Model file for the job. Use its own axes, mm. Face numbers are marked on the shaded views. Give positions to 0.01 mm unless a question says otherwise; leave off trailing zeros. Write each loop counter-clockwise with the first axis right and the second up, starting at its lowest first coordinate (ties: lowest second). Pieces come first, ordered by that corner, then holes.
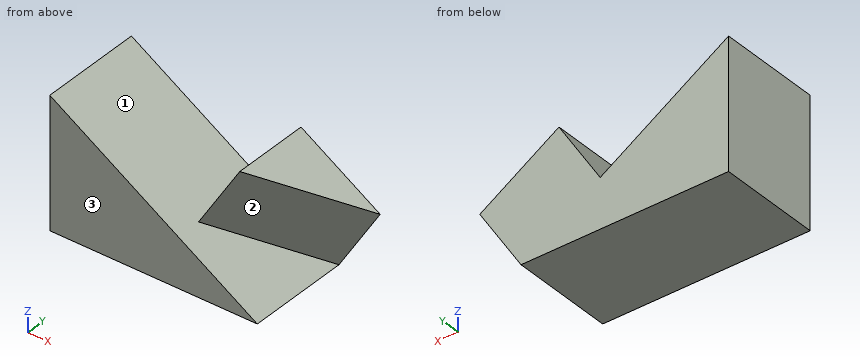
```python
from build123d import *

# Parameters (mm, degrees)
F1_DEPTH = 25.4
F3_DEPTH = 19.05


with BuildPart() as f1:
    # F0 (on Front) → F1 (new body)
    with BuildSketch(Plane.XZ):
        Polygon((0, 31.75), (0, 0), (50.8, 0), align=None)
    extrude(amount=F1_DEPTH)

    # F2 (on face) → F3 (join)
    with BuildSketch(Plane(origin=(14.2696629213, 0, 22.8314606742), x_dir=(0.847998304, 0, -0.52999894), z_dir=(0.52999894, 0, 0.847998304))):
        Polygon((20.2183138435, -19.05), (43.0783138435, 0), (20.2183138435, 0), align=None)
    extrude(amount=F3_DEPTH)


solid = f1.part
```
1. Probe probe 1 along X at (y, z) = (-5, 25.5); probe 2 along X at (y, z) = (-11.5, 16.5); probe 3 along Z at (x, y) = (14.5, -12). List the from-to ranges inside material, lowest first.
Calculated:
probe 1: x = 0 to 10, 39.78 to 45.94
probe 2: x = 0 to 24.4, 34.15 to 44.84
probe 3: z = 0 to 22.69
2. Slice it at A-A, the plane z = 23. Write the cut outline in (x, y), and give its area (3 significant figures).
Calculated:
outline: (0, -25.4) - (14, -25.4) - (14, 0) - (0, 0) - close; (38.22, -19.05) - (49.94, -10.76) - (49.94, 0) - (38.22, 0) - close
area: 530 mm2
3. Slice it at C-C, the plane x = 12. Write the cut outline in (y, z), and give its area (3 significant figures).
Calculated:
outline: (-25.4, 0) - (0, 0) - (0, 24.25) - (-25.4, 24.25) - close
area: 616 mm2
4. Pull direction X, two halves, no side cores. Call the marked faces 1, 2 and 3: +X half, -X half, draft (parallel to the pull), parting line (faces both ways), or undercut.
Calculated:
face 1: undercut
face 2: +X half
face 3: draft
5. Slice it at B-B, the plane y = -2.5. Write the cut outline in (x, z).
Calculated:
outline: (0, 0) - (50.8, 0) - (48.26, 1.59) - (58.35, 17.74) - (41.51, 28.27) - (31.41, 12.12) - (0, 31.75) - close
6. Pin check, flat tips, straight feed: P1, Ø1, axis at x = 23, z = 14, coming from the +Y side; P2, Ø8, axis at x = 50.5, y = -21.5, coming from the +Z side; P3, Ø8, axis at x = 45, z = 27, coming from the -Y side; P4, Ø3, axis at x = 29.5, y = -5.5, coming from the +Z side. Stop position of each tip, or through.
Calculated:
P1: stops at y = 0
P2: stops at z = 2.69
P3: stops at y = -19.05
P4: stops at z = 14.25
7. Slice it at D-D, the plane z = 10. Write the cut outline in (x, y).
Calculated:
outline: (0, -25.4) - (34.8, -25.4) - (34.8, -15.72) - (57.05, 0) - (0, 0) - close
